Build history of the part. All positions in model axes, mm. A direction names the side the tool comes from. Give positions to 0.01 mm unless a question says otherwise; leave off trailing zeros. Loops run counter-clockwise (first coordinate to the right, second up) from the corner with the lowest first, then second, coordinate; pieces in that order, holes last. Notation, with made-up numbers: (55.5, 76) -> (69.5, 76) arc R12 ccw to (69.5, 90) -> close; hole circle Ø2 at (66, 53). An arc over 180 degrees is marked (long way). One line per question, with ' | ' between items. Start each with the question number.
(1) Slice it at B-B, the plane z = 127. Write the cut outline in (x, y), then the cut area to 3 significant figures.
(2) Slice it at C-C, the plane z = 82. Write the cut outline in (x, y).
(3) Flat gauge pins, fed straight in: pin 1 Ø2 at (x, y) = (2.5, 27) entering from -Z; pin 2 Ø6 at (x, y) = (-31.5, 41) entering from +Z. Where does each tip first touch, or does it go through?
(4) Drill centre lines: L1, parallel to X at y = 15.5, z = 61.5; L2, parallel to Y at x = 74, z = 18; L3, parallel to X at y = -5, z = 143 (3 decimals). Where is each one in solid material? Low to high. Write a range as from..to.
(5) Mould opens along Y. For faces 6 (the face through (7.539, -4, 68)), 7 (the face through (3, -77.687, 75)), 8 (the face through (-30, -75, 153)) say: pulls with the +Y half, pulls with the -Y half, needs draft (parallel to the pull), parting line crosses it, or undercut.
(6) Slice it at A-A, the plane y = 0. Write the cut outline in (x, z).
(7) 3-axis set-ups, long thin cutter, end or side, ignore diameter. For faces 1 (the face through (105.4, 15.05, 139.07)), 2 (the face through (3, 69.147, 149)), 3 (the face through (5, -71.459, 80)), 4 (the face through (5, -60.822, 117)), 5 (the face through (-110.859, -4, 75)): which of +Z, -Z, +X, -X, +Y, -Y reach the whole face in a straight line?
(8) Slice it at D-D, the plane x = 61. Write the cut outline in (y, z), then the cut area to 3 significant figures.
```python
from build123d import *

# Parameters (mm, degrees)
SKETCH1_W           = 230
SKETCH1_H           = 150
BOSS_EXTRUDE1_DEPTH = 150
SKETCH2_R           = 50.188302383
SKETCH2_R_2         = 50.087955562
CUT_EXTRUDE1_DEPTH  = 27
SKETCH3_W           = 219.220450204
SKETCH3_H           = 138.871598106
CUT_EXTRUDE2_DEPTH  = 134
SKETCH4_W           = 230
SKETCH4_H           = 150
BOSS_EXTRUDE2_DEPTH = 3
SKETCH5_W           = 223.297854639
SKETCH5_H           = 143.428697179
CUT_EXTRUDE3_DEPTH  = 9
SKETCH7_W           = 5.736257362
SKETCH7_H           = 137.728394846
BOSS_EXTRUDE5_DEPTH = 110
SKETCH8_R           = 1.5
CUT_EXTRUDE4_DEPTH  = 10
SKETCH9_W           = 34.045014521
SKETCH9_H           = 115.879735823
CUT_EXTRUDE5_DEPTH  = 10


with BuildPart() as part:
    # Sketch1 → Boss-Extrude1 (new body)
    with BuildSketch(Plane.XY):
        with Locations((4.141274238, -2.686980609)):
            Rectangle(SKETCH1_W, SKETCH1_H)
    extrude(amount=BOSS_EXTRUDE1_DEPTH)

    # Sketch2 → Cut-Extrude1 (cut)
    with BuildSketch(Plane.XY.offset(150)):
        with Locations((-48.385288776, 0)):
            Circle(SKETCH2_R)
        with Locations((57.627226531, 0)):
            Circle(SKETCH2_R_2)
    extrude(amount=-CUT_EXTRUDE1_DEPTH, mode=Mode.SUBTRACT)

    # Sketch3 → Cut-Extrude2 (cut)
    with BuildSketch(Plane(origin=(0, 0, 0), x_dir=(-1, 0, 0), z_dir=(0, 0, -1))):
        with Locations((-4.141274238, -3.166675249)):
            Rectangle(SKETCH3_W, SKETCH3_H)
    extrude(amount=-CUT_EXTRUDE2_DEPTH, mode=Mode.SUBTRACT)

    # Sketch4 → Boss-Extrude2 (add)
    with BuildSketch(Plane.XY.offset(150)):
        with Locations((4.141274238, -2.686980609)):
            Rectangle(SKETCH4_W, SKETCH4_H)
    extrude(amount=BOSS_EXTRUDE2_DEPTH)

    # Sketch5 → Cut-Extrude3 (cut)
    with BuildSketch(Plane.XY.offset(153)):
        with Locations((4.740892538, -2.567056949)):
            Rectangle(SKETCH5_W, SKETCH5_H)
    extrude(amount=-CUT_EXTRUDE3_DEPTH, mode=Mode.SUBTRACT)

    # Sketch7 → Boss-Extrude5 (add)
    with BuildSketch(Plane(origin=(0, 0, 134), x_dir=(-1, 0, 0), z_dir=(0, 0, -1))):
        with Locations((-4.671142288, -2.595073619)):
            Rectangle(SKETCH7_W, SKETCH7_H)
    extrude(amount=BOSS_EXTRUDE5_DEPTH)

    # Sketch8 → Cut-Extrude4 (cut)
    with BuildSketch(Plane(origin=(0, 0, 0), x_dir=(-1, 0, 0), z_dir=(0, 0, -1))):
        with Locations((-116.215713327, 69.343694299)):
            Circle(SKETCH8_R)
        with Locations((108.173667939, -74.477152429)):
            Circle(SKETCH8_R)
    extrude(amount=-CUT_EXTRUDE4_DEPTH, mode=Mode.SUBTRACT)

    # Sketch9 → Cut-Extrude5 (cut)
    with BuildSketch(Plane(origin=(7.539270969, 0, 0), x_dir=(0, 0, -1), z_dir=(1, 0, 0))):
        with Locations((-116.97749274, -2.881933203)):
            Rectangle(SKETCH9_W, SKETCH9_H)
    extrude(amount=-CUT_EXTRUDE5_DEPTH, mode=Mode.SUBTRACT)


solid = part.part
```
Final values:
1) outline: (-110.86, -77.69) -> (119.14, -77.69) -> (119.14, 72.31) -> (-110.86, 72.31) -> close; (1.8, -71.46) -> (7.54, -71.46) -> (7.54, -60.82) -> (1.8, -60.82) -> close; hole (-105.47, -72.6) -> (113.75, -72.6) -> (113.75, 66.27) -> (7.54, 66.27) -> (7.54, 55.06) -> (1.8, 55.06) -> (1.8, 66.27) -> (-105.47, 66.27) -> close | area: 4,180 mm2
2) outline: (-110.86, -77.69) -> (119.14, -77.69) -> (119.14, 72.31) -> (-110.86, 72.31) -> close; hole (-105.47, -72.6) -> (113.75, -72.6) -> (113.75, 66.27) -> (7.54, 66.27) -> (7.54, -71.46) -> (1.8, -71.46) -> (1.8, 66.27) -> (-105.47, 66.27) -> close
3) pin 1: z = 24 | pin 2: through
4) L1: -110.86..-105.47, 1.8..7.54, 113.75..119.14 | L2: -77.69..-72.6, 66.27..72.31 | L3: -110.859..-98.324, 1.553..7.789, 107.465..119.141
5) face 6: undercut | face 7: pulls with the -Y half | face 8: needs draft
6) outline: (-110.86, 0) -> (-105.47, 0) -> (-105.47, 134) -> (-98.57, 134) -> (-98.57, 144) -> (-106.91, 144) -> (-106.91, 153) -> (-110.86, 153) -> close; (1.8, 24) -> (7.54, 24) -> (7.54, 99.95) -> (1.8, 99.95) -> close; (1.8, 134) -> (7.54, 134) -> (7.54, 144) -> (1.8, 144) -> close; (107.72, 134) -> (113.75, 134) -> (113.75, 0) -> (119.14, 0) -> (119.14, 153) -> (116.39, 153) -> (116.39, 144) -> (107.72, 144) -> close
7) face 1: +Z, -Z | face 2: +Z | face 3: -Z | face 4: none | face 5: +Z, -Z, -X, +Y, -Y
8) outline: (-77.69, 0) -> (-72.6, 0) -> (-72.6, 134) -> (-49.97, 134) -> (-49.97, 144) -> (-74.28, 144) -> (-74.28, 153) -> (-77.69, 153) -> close; (49.97, 134) -> (66.27, 134) -> (66.27, 0) -> (72.31, 0) -> (72.31, 153) -> (69.15, 153) -> (69.15, 144) -> (49.97, 144) -> close | area: 2,050 mm2
